Geometry: final body of the model. Coordinates: model frame, mm. Face numbers are marked on the shaded views. A direction names the side the tool comes from. Round coordinates to 2 decimals unless told otherwise and drop trailing zeros. Loops run counter-clockwise (first coordinate to the right, second up) from the corner with the lowest first, then second, coordinate; pieces in that order, holes last. Notation, with made-up numbers: (1.25, 81) -> (28.25, 81) arc R14 cw to (28.25, 108) -> close; hole circle Ø1 at (84, 80). An arc over 180 degrees is marked (long way). Answer in a Markdown table with one row per item.
```python
from build123d import *

# Parameters (mm, degrees)
SKETCH_1_R           = 10
EXTRUDE_1_DEPTH      = 200
EXTRUDE_2_DEPTH      = 15
EXTRUDE_2_DEPTH_BACK = 15
SKETCH_4_R           = 10
EXTRUDE_3_DEPTH      = 60


with BuildPart() as part:
    # Sketch 1 → Extrude 1 (new body)
    with BuildSketch(Plane(origin=(0, 0, 0), x_dir=(1, 0, 0), z_dir=(0, 1, 0))):
        with Locations(Location((0, 0, 0), (0, 0, 270))):
            Circle(SKETCH_1_R)
    extrude(amount=EXTRUDE_1_DEPTH)

    # Sketch 2 → Extrude 2 (add, two sides: drawn at the far end of the back side and taken through both)
    with BuildSketch(Plane(origin=(0, 0, 0), x_dir=(0, 0, -1), z_dir=(1, 0, 0)).offset(-EXTRUDE_2_DEPTH_BACK)):
        with BuildLine():
            Line((-10, 40), (10, 40))
            ThreePointArc((10, 40), (20.606601718, 35.606601718), (25, 25))
            Line((25, 25), (25, 15))
            ThreePointArc((25, 15), (20.606601718, 4.393398282), (10, 0))
            Line((10, 0), (-10, 0))
            ThreePointArc((-10, 0), (-20.606601718, 4.393398282), (-25, 15))
            Line((-25, 15), (-25, 25))
            ThreePointArc((-25, 25), (-20.606601718, 35.606601718), (-10, 40))
        make_face()
    extrude(amount=EXTRUDE_2_DEPTH + EXTRUDE_2_DEPTH_BACK)

    # Sketch 4 → Extrude 3 (add)
    with BuildSketch(Plane.ZY.offset(15)):
        with Locations((0, 15)):
            Circle(SKETCH_4_R)
    extrude(amount=EXTRUDE_3_DEPTH)


solid = part.part
```
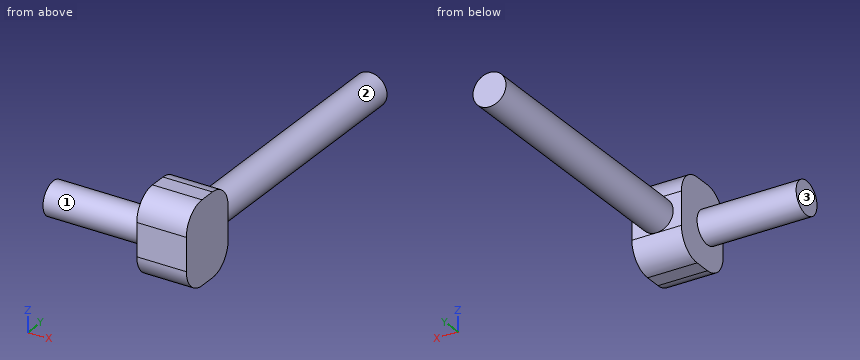
Item 1: Cut plane D-D (z = 13). Output: boundary loops of the cut face in (x, y).
Answer:
| item | result |
|---|---|
| outline | (-15, 0.3) -> (15, 0.3) -> (15, 39.7) -> (-15, 39.7) -> close |
Item 2: Reachability of the marked faces 1, 2 and 3 from +Z, -Z, +X, -X, +Y, -Y: full face, straight path, thin tool, end or side. Return the list, or none.
Answer:
| item | result |
|---|---|
| face 1 | -X |
| face 2 | +Y |
| face 3 | +Z, -Z, -X, +Y, -Y |
Item 3: Cut plane C-C (x = -39). Output: boundary loops of the cut face in (y, z).
Answer:
| item | result |
|---|---|
| outline | circle Ø20 at (15, 0) |
Item 4: Line query: probe 1 along Y at (x, z) = (-13.5, 4); probe 2 along X at (y, z) = (14.5, -21); probe 3 along Y at (x, z) = (-6, -13). Output: solid intervals per line, ascending. Write a range as [from, to].
Answer:
| item | result |
|---|---|
| probe 1 | y = [0, 40] |
| probe 2 | x = [-15, 15] |
| probe 3 | y = [0.3, 39.7] |
Item 5: Cut plane B-B (y = 63). Output: boundary loops of the cut face in (x, z).
Answer:
| item | result |
|---|---|
| outline | circle Ø20 at (0, 0) |
Item 6: Cut plane A-A (z = 0). Output: boundary loops of the cut face in (x, y).
Answer:
| item | result |
|---|---|
| outline | (-75, 5) -> (-15, 5) -> (-15, 0) -> (15, 0) -> (15, 40) -> (10, 40) -> (10, 200) -> (-10, 200) -> (-10, 40) -> (-15, 40) -> (-15, 25) -> (-75, 25) -> close |
Item 7: Pin query (flat end, axial travel): pin 1 Ø6 at (x, y) = (-11.5, 37.5) entering from -Z; pin 2 Ø6 at (x, z) = (-32.5, 2.5) entering from +Y; pin 3 Ø12 at (y, z) = (83, -18.5) entering from -X (1 decimal); pin 4 Ø1.5 at (x, z) = (-43.5, 2) entering from +Y. Return the tip coordinate at first contact, or that it passes through.
Answer:
| item | result |
|---|---|
| pin 1 | stops at z = -21.61 |
| pin 2 | stops at y = 25 |
| pin 3 | passes through |
| pin 4 | stops at y = 24.92 |
